from build123d import *

# Parameters (mm, degrees)
F1_DEPTH = 4.7625


with BuildPart() as f1:
    # F0 (on Front) → F1 (new body)
    with BuildSketch(Plane.XZ):
        with BuildLine():
            Line((76.2, 0), (0, 0))
            Line((0, 0), (0, -25.4))
            Line((0, -25.4), (19.05, -25.4))
            ThreePointArc((19.05, -25.4), (23.540128, -27.259872), (25.4, -31.75))
            Line((25.4, -31.75), (25.4, -76.2))
            Line((25.4, -76.2), (50.8, -76.2))
            Line((50.8, -76.2), (50.8, -31.75))
            ThreePointArc((50.8, -31.75), (52.659872, -27.259872), (57.15, -25.4))
            Line((57.15, -25.4), (76.2, -25.4))
            Line((76.2, -25.4), (76.2, 0))
        make_face()
    extrude(amount=F1_DEPTH)


solid = f1.part
Geometry: final body of the model. Coordinates: model frame, mm. A direction names the side the tool comes from. Give positions to 0.01 mm unless a question says otherwise; leave off trailing zeros. Order: outer loops, then holes, each group sorted by start corner. A loop starts at its lowest first (then second) coordinate and runs counter-clockwise, first axis right, second up. Notation, with made-up numbers: (32.5, -21.5) - (53.5, -21.5) arc R16 ccw to (53.5, -10.5) - close; hole circle Ø2 at (-35.75, 20.5). An arc over 180 degrees is marked (long way). Use CSV: the item, a comma, the result in double quotes.
1. Section query B-B (x = 10). Output: boundary loops of the cut face in (y, z).
Answers below:
outline,"(-4.76, -25.4) - (0, -25.4) - (0, 0) - (-4.76, 0) - close"
2. Section query A-A (y = -2). Output: boundary loops of the cut face in (x, z).
Answers below:
outline,"(0, -25.4) - (19.05, -25.4) arc R6.35 cw to (25.4, -31.75) - (25.4, -76.2) - (50.8, -76.2) - (50.8, -31.75) arc R6.35 cw to (57.15, -25.4) - (76.2, -25.4) - (76.2, 0) - (0, 0) - close"
3. Access query for faces 4 (the face through (9, -2, -25.4)), 5 (the face through (38, -2, -76.2)), 6 (the face through (50.8, -2, -54)). Directions: +Z, -Z, +X, -X, +Y, -Y. A direction counts if a zero-diameter tool reaches every point of the face in a straight line with its end or side. Return the directions, or none.
Answers below:
face 4,"-Z, -X, +Y, -Y"
face 5,"-Z, +X, -X, +Y, -Y"
face 6,"-Z, +X, +Y, -Y"
4. Mould query, pull axis Z, two halves, no side actions, for faces 1 (the face through (23.49, -2.35, -27.21)), 2 (the face through (39, -2, 0)), 3 (the face through (76.2, -2, -13)). Classes: +Z half, -Z half, draft (parallel to the pull), parting line (faces both ways), or undercut.
Answers below:
face 1,"-Z half"
face 2,"+Z half"
face 3,"draft"
5. Material intervals for line 1 along X through (y, z) = (-3, -73); line 2 along Z through (x, y) = (12, -1.2); line 3 along Z through (x, y) = (52, -2.4), sorted ascending. Write a range as from..to.
Answers below:
line 1,"25.4..50.8"
line 2,"-25.4..0"
line 3,"-28.04..0"
6. Contact query for flat-ended pins moving along their axis: pin 1 (1.4 mm diameter, centred on x = 9, y = -2, fed in from -Z); pin 2 (2 mm diameter, centred on y = -0.5, z = -55, fed in from -X). Output: stop coordinate, or through.
Answers below:
pin 1,"z = -25.4"
pin 2,"x = 25.4"
7. Section query C-C (z = -47). Output: boundary loops of the cut face in (x, y), plus the area to 3 significant figures.
Answers below:
outline,"(25.4, -4.76) - (50.8, -4.76) - (50.8, 0) - (25.4, 0) - close"
area,"121 mm2"
